Could you check a few things on this model? Use its own coordinates, in mm. Face numbers are marked on the shaded views. Coordinates: 2 decimals unless noted, no trailing zeros. Write each loop counter-clockwise with the first axis right and the second up, starting at its lowest first coordinate (ties: lowest second). Pieces come first, ordered by that corner, then holes.
Item 1: I want a section at A-A on x = 10. Please give me the cut outline in (y, z), then the cut area to 3 significant figures.
Item 2: I want a section at B-B on y = -199.5. Please give me the cut outline in (x, z), then the cut area to 3 significant figures.
Item 3: Thinking about a two-plate mould opening in X: for the marked faces 1, 2, 3 and 4, which applies, +X half, -X half, draft (parallel to the pull), parting line (faces both ways), or undercut?
Item 4: I want a section at C-C on z = -1.5. Please give me the cut outline in (x, y), then the cut area to 3 significant figures.
Item 5: If I drill on probe 1 along X at (y, z) = (-75, 0.5); probe 2 along Z at (x, y) = (-8.5, -212.5); probe 3 along X at (y, z) = (-158, -11), over which ranges is the centre line in solid material (lowest first)?
from build123d import *

# Parameters (mm, degrees)
F0_W     = 50.8
F0_H     = 25.4
F1_DEPTH = 254
F2_W     = 47.6504
F2_H     = 22.2504
F3_DEPTH = 254
F4_R     = 1.524
F5_R     = 0.254


with BuildPart() as f1:
    # F0 (on Front) → F1 (new body)
    with BuildSketch(Plane.XZ):
        Rectangle(F0_W, F0_H)
    extrude(amount=F1_DEPTH)

    # F2 (on face) → F3 (cut, through all)
    with BuildSketch(Plane.XZ.offset(254)):
        Rectangle(F2_W, F2_H)
    extrude(amount=-F3_DEPTH, mode=Mode.SUBTRACT)

    # F4
    f4_edges = [f1.edges().sort_by_distance(p)[0] for p in [
        (23.8252, -127, -11.1252),
        (23.8252, -127, 11.1252),
        (-23.8252, -127, -11.1252),
        (-23.8252, -127, 11.1252),
    ]]
    fillet(f4_edges, radius=F4_R)

    # F5
    f5_edges = [f1.edges().sort_by_distance(p)[0] for p in [
        (-25.4, -127, 12.7),
        (25.4, -127, 12.7),
        (25.4, -127, -12.7),
        (-25.4, -127, -12.7),
    ]]
    fillet(f5_edges, radius=F5_R)


solid = f1.part
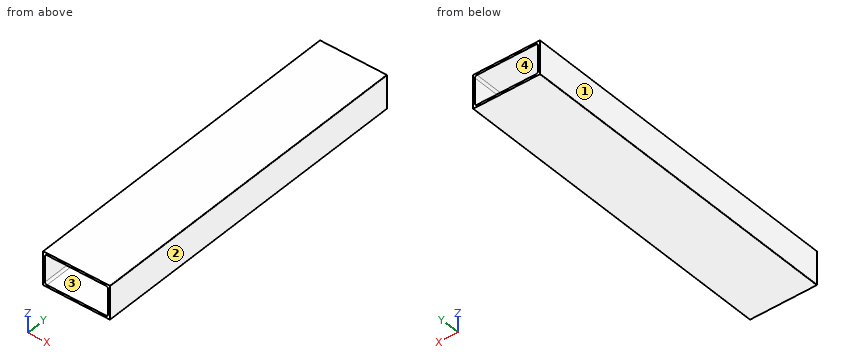
Response values:
1. outline: (-254, -12.7) - (0, -12.7) - (0, -11.13) - (-254, -11.13) - close; (-254, 11.13) - (0, 11.13) - (0, 12.7) - (-254, 12.7) - close
1. area: 800 mm2
2. outline: (-25.4, -12.45) arc R0.25 ccw to (-25.15, -12.7) - (25.15, -12.7) arc R0.25 ccw to (25.4, -12.45) - (25.4, 12.45) arc R0.25 ccw to (25.15, 12.7) - (-25.15, 12.7) arc R0.25 ccw to (-25.4, 12.45) - close; hole (-23.83, -9.6) arc R1.52 ccw to (-22.3, -11.13) - (22.3, -11.13) arc R1.52 ccw to (23.83, -9.6) - (23.83, 9.6) arc R1.52 ccw to (22.3, 11.13) - (-22.3, 11.13) arc R1.52 ccw to (-23.83, 9.6) - close
2. area: 232 mm2
3. face 1: -X half
3. face 2: +X half
3. face 3: undercut
3. face 4: undercut
4. outline: (-25.4, -254) - (-23.83, -254) - (-23.83, 0) - (-25.4, 0) - close; (23.83, -254) - (25.4, -254) - (25.4, 0) - (23.83, 0) - close
4. area: 800 mm2
5. probe 1: x = -25.4 to -23.83, 23.83 to 25.4
5. probe 2: z = -12.7 to -11.13, 11.13 to 12.7
5. probe 3: x = -25.4 to -22.91, 22.91 to 25.4
